```python
from build123d import *

# Parameters (mm, degrees)
SKETCH3_R                                         = 50
SKETCH3_R_2                                       = 12.7
BOSS_EXTRUDE4_DEPTH                               = 4.5
CUT_EXTRUDE18_DEPTH                               = 10
FILLET2_R                                         = 0.5
CSK_FOR_4_FLAT_HEAD_MACHINE_SCREW_100_D           = 3.4544
CSK_FOR_4_FLAT_HEAD_MACHINE_SCREW_100_CSINK_D     = 5.715
CSK_FOR_4_FLAT_HEAD_MACHINE_SCREW_100_CSINK_ANGLE = 100


with BuildPart() as part:
    # Sketch3 → Boss-Extrude4 (new body)
    with BuildSketch(Plane(origin=(0, 0, 0), x_dir=(1, 0, 0), z_dir=(0, 1, 0))):
        Circle(SKETCH3_R)
        Circle(SKETCH3_R_2, mode=Mode.SUBTRACT)
    extrude(amount=BOSS_EXTRUDE4_DEPTH)

    # Sketch6 → Cut-Extrude18 (cut)
    with BuildSketch(Plane(origin=(0, 0, 0), x_dir=(1, 0, 0), z_dir=(0, 1, 0))):
        with BuildLine():
            Line((-38, -4.5), (-65, -4.5))
            Line((-65, -4.5), (-65, 4.5))
            Line((-65, 4.5), (-38, 4.5))
            ThreePointArc((-38, 4.5), (-35.878679656, 3.621320344), (-35, 1.5))
            Line((-35, 1.5), (-35, -1.5))
            ThreePointArc((-35, -1.5), (-35.878679656, -3.621320344), (-38, -4.5))
        make_face()
        with BuildLine():
            Line((-4.5, 38), (-4.5, 65))
            Line((-4.5, 65), (4.5, 65))
            Line((4.5, 65), (4.5, 38))
            ThreePointArc((4.5, 38), (3.621320344, 35.878679656), (1.5, 35))
            Line((1.5, 35), (-1.5, 35))
            ThreePointArc((-1.5, 35), (-3.621320344, 35.878679656), (-4.5, 38))
        make_face()
        with BuildLine():
            Line((38, 4.5), (65, 4.5))
            Line((65, 4.5), (65, -4.5))
            Line((65, -4.5), (38, -4.5))
            ThreePointArc((38, -4.5), (35.878679656, -3.621320344), (35, -1.5))
            Line((35, -1.5), (35, 1.5))
            ThreePointArc((35, 1.5), (35.878679656, 3.621320344), (38, 4.5))
        make_face()
        with BuildLine():
            Line((4.5, -38), (4.5, -65))
            Line((4.5, -65), (-4.5, -65))
            Line((-4.5, -65), (-4.5, -38))
            ThreePointArc((-4.5, -38), (-3.621320344, -35.878679656), (-1.5, -35))
            Line((-1.5, -35), (1.5, -35))
            ThreePointArc((1.5, -35), (3.621320344, -35.878679656), (4.5, -38))
        make_face()
    extrude(amount=CUT_EXTRUDE18_DEPTH, mode=Mode.SUBTRACT)

    # Fillet2
    fillet2_edges = [part.edges().sort_by_distance(p)[0] for p in [
        (-49.797088268, 2.25, -4.5),
        (-49.797088268, 2.25, 4.5),
        (4.5, 2.25, -49.797088268),
        (-4.5, 2.25, -49.797088268),
        (49.797088268, 2.25, 4.5),
        (49.797088268, 2.25, -4.5),
        (-4.5, 2.25, 49.797088268),
        (4.5, 2.25, 49.797088268),
    ]]
    fillet(fillet2_edges, radius=FILLET2_R)

    # CSK for #4 Flat Head Machine Screw (100)1 (through all)
    with Locations(Plane(origin=(0, 4.5, 0), x_dir=(1, 0, 0), z_dir=(0, 1, 0))):
        with Locations((0, -16.862709614), (0, 16.862709614)):
            CounterSinkHole(CSK_FOR_4_FLAT_HEAD_MACHINE_SCREW_100_D / 2, CSK_FOR_4_FLAT_HEAD_MACHINE_SCREW_100_CSINK_D / 2, counter_sink_angle=CSK_FOR_4_FLAT_HEAD_MACHINE_SCREW_100_CSINK_ANGLE)


solid = part.part
```
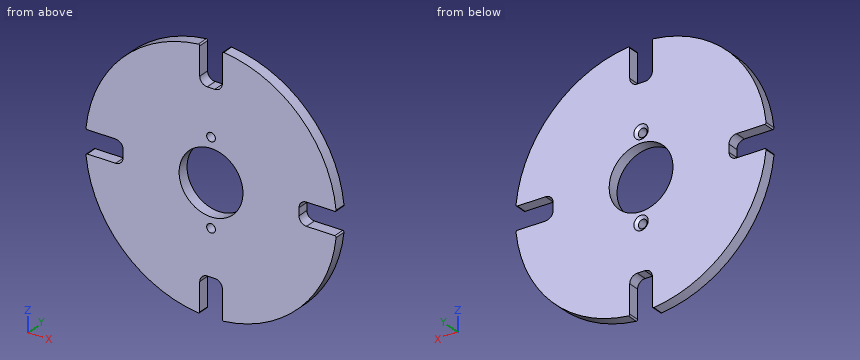
Can you work these out from the model? Positions are in its coordinate system, mm. Give positions to 0.01 mm unless a question says otherwise; leave off trailing zeros. Write each loop counter-clockwise with the first axis right and the second up, starting at its lowest first coordinate (ties: lowest second). Pieces come first, ordered by that corner, then holes. Notation, with made-up numbers: (3.5, 24) - (13.5, 24) arc R9 cw to (13.5, 37) - close; hole circle Ø3 at (49, -28.75). An arc over 180 degrees is marked (long way). Write item = value, one per line. Start each with the question number.
1. Imagine slicing it at A-A (x = 0). Please give me the cut outline in (y, z), and give its area (3 significant figures).
2. Please list where these lines run through material, in increasing order: line 1 (Z direction, x = 0, y = 3.5); line 2 (X direction, y = 0.4, z = 39); line 3 (X direction, y = 3.4, z = 0).
3. Imagine slicing it at C-C (z = -11). Please give me the cut outline in (x, y) (3 decimals).
4. Imagine slicing it at B-B (z = 0). Please give me the cut outline in (x, y).
5. For pin 1 (2 mm diameter, centred on y = 2, z = -46, fed in from +X); pin 2 (2 mm diameter, centred on x = 0, z = 16.86, fed in from -Y); pin 3 (1.5 mm diameter, centred on y = 3, z = 21, fed in from +X); pin 4 (2 mm diameter, centred on y = 2.5, z = 45, fed in from -X), each with a flat end and sliding along its axis, tell me the tip position at first contact or that it passes through.
6. Imagine slicing it at D-D (y = 1.1). Count the separate pieces of the cut face and the enclosed holes in it, and give its area (3 significant figures).
Worked answers:
q1.outline = (0, -35) - (4.5, -35) - (4.5, -19.72) - (3.55, -18.59) - (0, -18.59) - close; (0, -15.14) - (3.55, -15.14) - (4.5, -14.01) - (4.5, -12.7) - (0, -12.7) - close; (0, 12.7) - (4.5, 12.7) - (4.5, 14.01) - (3.55, 15.14) - (0, 15.14) - close; (0, 18.59) - (3.55, 18.59) - (4.5, 19.72) - (4.5, 35) - (0, 35) - close
q1.area = 167 mm2
q2.line_1 = -35 to -18.59, -15.14 to -12.7, 12.7 to 15.14, 18.59 to 35
q2.line_2 = -31.29 to -4.5, 4.5 to 31.29
q2.line_3 = -35 to -12.7, 12.7 to 35
q3.outline = (-48.775, 0) - (-6.347, 0) - (-6.347, 4.5) - (-48.775, 4.5) - close; (6.347, 0) - (48.775, 0) - (48.775, 4.5) - (6.347, 4.5) - close
q4.outline = (-35, 0) - (-12.7, 0) - (-12.7, 4.5) - (-35, 4.5) - close; (12.7, 0) - (35, 0) - (35, 4.5) - (12.7, 4.5) - close
q5.pin_1 = 21.79
q5.pin_2 = through
q5.pin_3 = 45.72
q5.pin_4 = -23.75
q6.separate_pieces = 1
q6.enclosed_holes = 3
q6.area = 6,810 mm2
